CAD build for the part. Positions are in the model's coordinates, mm. A direction names the side the tool comes from. Give positions to 0.01 mm unless a question says otherwise; leave off trailing zeros. Loops run counter-clockwise (first coordinate to the right, second up) from the corner with the lowest first, then second, coordinate; pieces in that order, holes last. Notation, with made-up numbers: (41.25, 22) - (83.25, 22) arc R16 ccw to (83.25, 29) - close; hole circle Ø1 at (72.25, 82.25). An arc over 180 degrees is marked (long way). Return JSON: item names as keys, results as strings.
from build123d import *

# Parameters (mm, degrees)
F0_R     = 165.1
F1_DEPTH = 381
F2_R     = 146.05
F3_DEPTH = 330.2
F4_W     = 254
F4_H     = 76.2
F5_DEPTH = 177.8
F7_DEPTH = 25.4


with BuildPart() as f1:
    # F0 (on Top) → F1 (new body)
    with BuildSketch(Plane.XY):
        Circle(F0_R)
    extrude(amount=F1_DEPTH)

    # F2 (on face) → F3 (cut)
    with BuildSketch(Plane.XY.offset(381)):
        Circle(F2_R)
    extrude(amount=-F3_DEPTH, mode=Mode.SUBTRACT)

    # F4 (on Front) → F5 (cut)
    with BuildSketch(Plane.XZ):
        with Locations((0, 88.9)):
            Rectangle(F4_W, F4_H)
    extrude(amount=F5_DEPTH, mode=Mode.SUBTRACT)

    # F6 (on face) → F7 (cut)
    with BuildSketch(Plane.XY.offset(381)):
        with BuildLine():
            ThreePointArc((12.7, 164.6108137396), (6.3547089469, 164.9776581062), (0, 165.1))
            ThreePointArc((0, 165.1), (-6.3547089469, 164.9776581062), (-12.7, 164.6108137396))
            Line((-12.7, 164.6108137396), (-12.7, 145.4967783148))
            ThreePointArc((-12.7, 145.4967783148), (0, 146.05), (12.7, 145.4967783148))
            Line((12.7, 145.4967783148), (12.7, 164.6108137396))
        make_face()
        with BuildLine():
            Line((-145.4967783148, 12.7), (-164.6108137396, 12.7))
            ThreePointArc((-164.6108137396, 12.7), (-164.9776581062, 6.3547089469), (-165.1, 0))
            ThreePointArc((-165.1, 0), (-164.9776581062, -6.3547089469), (-164.6108137396, -12.7))
            Line((-164.6108137396, -12.7), (-145.4967783148, -12.7))
            ThreePointArc((-145.4967783148, -12.7), (-146.05, 0), (-145.4967783148, 12.7))
        make_face()
        with BuildLine():
            ThreePointArc((12.7, -145.4967783148), (0, -146.05), (-12.7, -145.4967783148))
            Line((-12.7, -145.4967783148), (-12.7, -164.6108137396))
            ThreePointArc((-12.7, -164.6108137396), (-6.3547090887, -164.9776581007), (-2.839e-07, -165.1))
            ThreePointArc((-2.839e-07, -165.1), (6.354708805, -164.9776581116), (12.7, -164.6108137396))
            Line((12.7, -164.6108137396), (12.7, -145.4967783148))
        make_face()
        with BuildLine():
            ThreePointArc((165.1, 0), (164.9776581062, 6.3547089469), (164.6108137396, 12.7))
            Line((164.6108137396, 12.7), (145.4967783148, 12.7))
            ThreePointArc((145.4967783148, 12.7), (145.9116290309, 6.3560218343), (146.05, 0))
            ThreePointArc((146.05, 0), (145.9116290309, -6.3560218343), (145.4967783148, -12.7))
            Line((145.4967783148, -12.7), (164.6108137396, -12.7))
            ThreePointArc((164.6108137396, -12.7), (164.9776581062, -6.3547089469), (165.1, 0))
        make_face()
    extrude(amount=-F7_DEPTH, mode=Mode.SUBTRACT)


solid = f1.part
1. Cut at C-C, the plane y = -116. Write the cut outline in (x, z), plus the area to 3 significant figures.
Values follow:
{"outline": "(-117.48, 0) - (117.48, 0) - (117.48, 50.8) - (-117.48, 50.8) - close; (-117.48, 127) - (-88.74, 127) - (-88.74, 381) - (-117.48, 381) - close; (88.74, 127) - (117.48, 127) - (117.48, 381) - (88.74, 381) - close", "area": "26,500 mm²"}
2. Drop flat-ended pins along their axis: P1, Ø9.5, axis at y = 156, z = 369.5, coming from the +X side; P2, Ø5.5, axis at y = 152.5, z = 367, coming from the -X side; P3, Ø4, axis at x = 69.5, z = 55.5, coming from the -Y side. Give the stop position or say it passes through.
Values follow:
{"P1": "stops at x = 66.19", "P2": "stops at x = -69.52", "P3": "stops at y = 127.35"}
3. Which spindle directions (+Z, -Z, +X, -X, +Y, -Y) get a long thin tool onto all of the face, cutting with end or side? Do faces 1 (the face through (-106, 106, 381)), 2 (the face through (155, -12.7, 368)), 3 (the face through (0, -155, 355.6)), 4 (the face through (-127, -89, 88)). Say none if no direction does.
Values follow:
{"face 1": "+Z, +X, -X, +Y, -Y", "face 2": "+Z, +X, -X", "face 3": "+Z, +Y, -Y", "face 4": "-Y"}
4. Drill centre lines: probe 1 along Y at (x, z) = (0, 302); probe 2 along Z at (x, y) = (100.5, -120); probe 3 along Z at (x, y) = (144.5, 19). Where is each one in solid material? Low to high.
Values follow:
{"probe 1": "y = -165.1 to -146.05, 146.05 to 165.1", "probe 2": "z = 0 to 50.8, 127 to 381", "probe 3": "z = 0 to 50.8"}
5. Cut at B-B, the plane y = 0. Write the cut outline in (x, z), plus the area to 3 significant figures.
Values follow:
{"outline": "(-165.1, 0) - (165.1, 0) - (165.1, 355.6) - (146.05, 355.6) - (146.05, 50.8) - (-146.05, 50.8) - (-146.05, 355.6) - (-165.1, 355.6) - close", "area": "28,400 mm²"}
6. Cut at D-D, the plane z = 152. Write the cut outline in (x, y), plus the area to 3 significant figures.
Values follow:
{"outline": "circle Ø330.2 at (0, 0); hole circle Ø292.1 at (0, 0)", "area": "18,600 mm²"}
7. Cut at A-A, the plane x = 0. Write the cut outline in (y, z), plus the area to 3 significant figures.
Values follow:
{"outline": "(-165.1, 0) - (165.1, 0) - (165.1, 355.6) - (146.05, 355.6) - (146.05, 50.8) - (-165.1, 50.8) - close; (-165.1, 127) - (-146.05, 127) - (-146.05, 355.6) - (-165.1, 355.6) - close", "area": "26,900 mm²"}
8. Pull direction X, two halves, no side cores. Call faces 5 (the face through (12.7, -155, 368)), 6 (the face through (155, 12.7, 368)): +X half, -X half, draft (parallel to the pull), parting line (faces both ways), or undercut.
Values follow:
{"face 5": "undercut", "face 6": "draft"}
